The model under review builds one solid part; all positions refer to its coordinate system, in mm. A direction names the side the tool comes from. Coordinates: 2 decimals unless noted, no trailing zeros. Write each loop counter-clockwise with the first axis right and the second up, starting at its lowest first coordinate (ties: lowest second). Pieces come first, ordered by that corner, then holes.
```python
from build123d import *

# Parameters (mm, degrees)
SKETCH1_R           = 10.5
SKETCH1_R_2         = 1.25
BOSS_EXTRUDE1_DEPTH = 4.5
SKETCH2_W           = 5
SKETCH2_H           = 40
BOSS_EXTRUDE2_DEPTH = 87.869807
SKETCH3_R           = 2.5
CUT_EXTRUDE1_DEPTH  = 6
BOSS_EXTRUDE3_DEPTH = 20
SKETCH5_W           = 12
SKETCH5_H           = 34
CUT_EXTRUDE2_DEPTH  = 87.869807
FILLET1_R           = 5


with BuildPart() as part:
    # Sketch1 → Boss-Extrude1 (new body)
    with BuildSketch(Plane.XY):
        Polygon((-26, -6), (0, -6), (13.72, -6), (13.72, 34), (0, 34), (-26, 34), align=None)
        with Locations((-13, 14)):
            Circle(SKETCH1_R, mode=Mode.SUBTRACT)
        with Locations((-3.9, 3.85)):
            Circle(SKETCH1_R_2, mode=Mode.SUBTRACT)
        with Locations((-23.05, 3.75)):
            Circle(SKETCH1_R_2, mode=Mode.SUBTRACT)
        with Locations((-22.85, 22.95)):
            Circle(SKETCH1_R_2, mode=Mode.SUBTRACT)
        with Locations((-3.7, 22.65)):
            Circle(SKETCH1_R_2, mode=Mode.SUBTRACT)
    extrude(amount=BOSS_EXTRUDE1_DEPTH)

    # Sketch2 → Boss-Extrude2 (add)
    with BuildSketch(Plane(origin=(0, 0, 0), x_dir=(-1, 0, 0), z_dir=(0, 0, -1))):
        with Locations((-11.22, 14)):
            Rectangle(SKETCH2_W, SKETCH2_H)
    extrude(amount=BOSS_EXTRUDE2_DEPTH)

    # Sketch3 → Cut-Extrude1 (cut, through all)
    with BuildSketch(Plane.ZY.offset(-8.72)):
        with Locations((-77.869807398, 29)):
            Circle(SKETCH3_R)
        with Locations((-77.869807398, -1)):
            Circle(SKETCH3_R)
        with Locations((-17.609807398, -1)):
            Circle(SKETCH3_R)
        with Locations((-17.609807398, 29)):
            Circle(SKETCH3_R)
    extrude(amount=-CUT_EXTRUDE1_DEPTH, mode=Mode.SUBTRACT)

    # Sketch4 → Boss-Extrude3 (add, symmetric)
    with BuildSketch(Plane(origin=(0, 14, 0), x_dir=(1, 0, 0), z_dir=(0, 1, 0))):
        Polygon((8.72, 13), (-3.28, 0), (8.72, 0), align=None)
    extrude(amount=BOSS_EXTRUDE3_DEPTH, both=True)

    # Sketch5 → Cut-Extrude2 (cut)
    with BuildSketch(Plane(origin=(0, 0, 0), x_dir=(-1, 0, 0), z_dir=(0, 0, -1))):
        with Locations((-2.72, 14)):
            Rectangle(SKETCH5_W, SKETCH5_H)
    extrude(amount=CUT_EXTRUDE2_DEPTH, mode=Mode.SUBTRACT)

    # Fillet1
    fillet1_edges = [part.edges().sort_by_distance(p)[0] for p in [
        (8.72, 14, 0),
    ]]
    fillet(fillet1_edges, radius=FILLET1_R)


solid = part.part
```
Item 1: To check wall thickness, follow line 1 along X through (y, z) = (3, 1); line 2 along X through (y, z) = (22, 1); line 3 along Y through (x, z) = (-3.9, 2.95). State the ranges of each line that lie inside material, in increasing order.
Solved:
line 1: x = -26 to -24.05, -22.05 to -4.82, -2.98 to 13.72
line 2: x = -26 to -23.66, -22.04 to -19.8, -6.2 to -4.77, -2.63 to 13.72
line 3: y = -6 to 2.6, 5.1 to 8.76, 19.24 to 21.42, 23.88 to 34
Item 2: Take a section at D-D, the plane x = -9. Write out the cut boundary in (y, z), plus the area to 3 significant figures.
Solved:
outline: (-6, 0) - (4.29, 0) - (4.29, 4.5) - (-6, 4.5) - close; (23.71, 0) - (34, 0) - (34, 4.5) - (23.71, 4.5) - close
area: 92.6 mm2
Item 3: Take a section at A-A, the plane y = 29. Write out the cut boundary in (x, z).
Solved:
outline: (-26, 0) - (3.72, 0) arc R5 cw to (8.72, -5) - (8.72, -15.11) - (13.72, -15.11) - (13.72, 4.5) - (-26, 4.5) - close; (8.72, -87.87) - (13.72, -87.87) - (13.72, -80.37) - (8.72, -80.37) - close; (8.72, -75.37) - (13.72, -75.37) - (13.72, -20.11) - (8.72, -20.11) - close
Item 4: For pin 1 (3 mm diameter, centred on x = -23.05, y = 3.75, fed in from -Z); pin 2 (4.5 mm diameter, centred on y = 29, z = -77.87, fed in from -X); pin 3 (10 mm diameter, centred on y = -2, z = -30.5, fed in from -X), all flat-tipped, find the tip position at first contact; note any pin that passes through.
Solved:
pin 1: stops at z = 0
pin 2: passes through
pin 3: stops at x = 8.72
Item 5: Machinability: for faces 4 (the face through (4, -3, -5)), 5 (the face through (-4.621, 23.495, 2.218)), which of the approach directions +Z, -Z, +X, -X, +Y, -Y give a long, thin tool a straight path to every point of the face, cutting with its end or side? Answer none if there is none.
Solved:
face 4: -Z, -X
face 5: +Z, -Z
Item 6: Take a section at C-C, the plane z = -11. Write out the cut boundary in (x, y).
Solved:
outline: (6.87, -6) - (13.72, -6) - (13.72, 34) - (6.87, 34) - (6.87, 31) - (8.72, 31) - (8.72, -3) - (6.87, -3) - close
Item 7: Take a section at B-B, the plane x = -13. Write out the cut boundary in (y, z), plus the area to 3 significant figures.
Solved:
outline: (-6, 0) - (3.5, 0) - (3.5, 4.5) - (-6, 4.5) - close; (24.5, 0) - (34, 0) - (34, 4.5) - (24.5, 4.5) - close
area: 85.5 mm2
Item 8: Mouldability with a two-part tool opening along Z and no side actions: class faces 1 (the face through (2.804, 32.521, -6.591)), 2 (the face through (-26, 14, 2)), 3 (the face through (11.18, 31.11, -16.27)) as pulls with the +Z half, pulls with the -Z half, needs draft (parallel to the pull), parting line crosses it, or undercut.
Solved:
face 1: pulls with the -Z half
face 2: needs draft
face 3: undercut
